```python
from build123d import *

# Parameters (mm, degrees)
SKETCH1_R           = 1.3251
SKETCH1_R_2         = 1.5002
BOSS_EXTRUDE1_DEPTH = 3.175


with BuildPart() as part:
    # Sketch1 → Boss-Extrude1 (new body)
    with BuildSketch(Plane(origin=(0, 0, 0), x_dir=(1, 0, 0), z_dir=(0, 1, 0))):
        with BuildLine():
            Line((24.252360584, 153.047337226), (24.066660584, 153.037137226))
            Line((24.066660584, 153.037137226), (41.780860584, 153.037137226))
            Line((41.780860584, 153.037137226), (41.780860584, 153.047237226))
            add(Edge.make_bspline(
                [(41.780860584, 153.047237226), (46.472460584, 153.023637226), (46.937960584, 158.355437226), (44.801360584, 160.253637226)],
                knots=[0.3, 0.3, 0.3, 0.3, 0.4, 0.4, 0.4, 0.4], degree=3))
            add(Edge.make_bspline(
                [(44.801360584, 160.253637226), (44.076060584, 160.918437226), (43.092260584, 161.292037226), (42.066560584, 161.292037226)],
                knots=[0.4, 0.4, 0.4, 0.4, 0.5, 0.5, 0.5, 0.5], degree=3))
            add(Edge.make_bspline(
                [(42.066560584, 161.292037226), (35.872760584, 161.305437226), (39.575560584, 167.746037226), (34.122660584, 167.769037226)],
                knots=[0.5, 0.5, 0.5, 0.5, 0.6, 0.6, 0.6, 0.6], degree=3))
            add(Edge.make_bspline(
                [(34.122660584, 167.769037226), (31.657460584, 167.779437226), (28.361660584, 167.993537226), (23.966660584, 167.746037226)],
                knots=[0.6, 0.6, 0.6, 0.6, 0.7, 0.7, 0.7, 0.7], degree=3))
            add(Edge.make_bspline(
                [(23.966660584, 167.746037226), (22.940960584, 167.746037226), (21.957160584, 167.079937226), (21.231860584, 165.894837226)],
                knots=[0.7, 0.7, 0.7, 0.7, 0.8, 0.8, 0.8, 0.8], degree=3))
            add(Edge.make_bspline(
                [(21.231860584, 165.894837226), (19.095260584, 162.510837226), (19.560760584, 153.005437226), (24.252360584, 153.047337226)],
                knots=[0.8, 0.8, 0.8, 0.8, 1, 1, 1, 1], degree=3))
        make_face()
        with Locations(Location((23.966660584, 157.037137226, 0), (0, 0, 270))):
            Circle(SKETCH1_R, mode=Mode.SUBTRACT)
        with Locations(Location((42.066460584, 157.037137226, 0), (0, 0, 270))):
            Circle(SKETCH1_R_2, mode=Mode.SUBTRACT)
    extrude(amount=BOSS_EXTRUDE1_DEPTH)


solid = part.part
```
Geometry: final body of the model. Coordinates: model frame, mm. Coordinates: 2 decimals unless noted, no trailing zeros. Answer as CSV lines item,"result". Start each with the question number.
Q1. Mould query, pull axis Z, two halves, no side actions, for faces 1 (the flat face through (33, 2, -153.037)), 2 (the flat face through (33, 3.175, -161)), 3 (the cylindrical face through (24.36, 1.57, -155.77)). Classes: released by +Z, released by -Z, zero draft, split by the parting line, or undercut.
Q2. Line query: line 1 (X direction, y = 0.95, z = -156.25); line 2 (X direction, y = 2.5, z = -156.5); line 3 (Z direction, x = 29.25, y = 0.4). Output: solid intervals per line, ascending. Write a range as from..to.
Q3. Pin query (flat end, axial travel): P1, Ø1.5, axis at x = 40, y = 2, coming from the -Z side; P2, Ø1.5, axis at x = 25, y = 2, coming from the -Z side. Return the tip coordinate at first contact, or that it passes through.
Q4. Cut plane A-A on z = -157. Count the separate pieces of the cut face and the enclosed holes in it, then the cut area to 3 significant figures.
Findings below:
1,face 1,"released by +Z"
1,face 2,"zero draft"
1,face 3,"undercut"
2,line 1,"x = 20.65..22.9, 25.03..40.79, 43.34..45.93"
2,line 2,"x = 20.57..22.76, 25.18..40.67, 43.47..45.97"
2,line 3,"z = -167.86..-153.04"
3,P1,"stops at z = -162.07"
3,P2,"stops at z = -167.82"
4,separate pieces,"3"
4,enclosed holes,"0"
4,area,"63.3 mm2"
